```python
from build123d import *

# Parameters (mm, degrees)
SALIENTE_EXTRUIR1_DEPTH = 19.65
CROQUIS2_R              = 2.575
CORTAR_EXTRUIR1_DEPTH   = 8.65


with BuildPart() as part:
    # Croquis1 → Saliente-Extruir1 (new body)
    with BuildSketch(Plane(origin=(0, 0, 0), x_dir=(1, 0, 0), z_dir=(0, 1, 0))):
        with BuildLine():
            Line((-5.5, 9.825), (5.5, 9.825))
            ThreePointArc((5.5, 9.825), (6.207106781, 9.532106781), (6.5, 8.825))
            Line((6.5, 8.825), (6.5, -8.825))
            ThreePointArc((6.5, -8.825), (6.207106781, -9.532106781), (5.5, -9.825))
            Line((5.5, -9.825), (-5.5, -9.825))
            ThreePointArc((-5.5, -9.825), (-6.207106781, -9.532106781), (-6.5, -8.825))
            Line((-6.5, -8.825), (-6.5, 8.825))
            ThreePointArc((-6.5, 8.825), (-6.207106781, 9.532106781), (-5.5, 9.825))
        make_face()
        with BuildLine():
            Line((-4.75, -6.825), (4.75, -6.825))
            ThreePointArc((4.75, -6.825), (4.926776695, -6.751776695), (5, -6.575))
            Line((5, -6.575), (5, 7.325))
            ThreePointArc((5, 7.325), (4.707106781, 8.032106781), (4, 8.325))
            Line((4, 8.325), (-4, 8.325))
            ThreePointArc((-4, 8.325), (-4.707106781, 8.032106781), (-5, 7.325))
            Line((-5, 7.325), (-5, -6.575))
            ThreePointArc((-5, -6.575), (-4.926776695, -6.751776695), (-4.75, -6.825))
        make_face(mode=Mode.SUBTRACT)
    extrude(amount=-SALIENTE_EXTRUIR1_DEPTH)

    # Croquis2 → Cortar-Extruir1 (cut)
    with BuildSketch(Plane.XY.offset(9.825)):
        with Locations((0, -4.65)):
            Circle(CROQUIS2_R)
        with Locations((0, -15)):
            Circle(CROQUIS2_R)
    extrude(amount=-CORTAR_EXTRUIR1_DEPTH, mode=Mode.SUBTRACT)


solid = part.part
```
The listing builds one solid part. Answer for the finished solid, in the listing's coordinates (mm). A direction names the side the tool comes from. Round coordinates to 2 decimals unless told otherwise and drop trailing zeros. Loops run counter-clockwise (first coordinate to the right, second up) from the corner with the lowest first, then second, coordinate; pieces in that order, holes last. Notation, with made-up numbers: (-32.75, 69.25) -> (0.25, 69.25) arc R12 ccw to (0.25, 90.25) -> close; hole circle Ø3 at (15.25, 81). An arc over 180 degrees is marked (long way). Use one line per item in the form item = value.
1. The part is cut by section D-D on y = -15. Determine the outline of the cut face in (x, z) (3 decimals).
Answer key:
outline = (-6.5, -8.825) arc R1 ccw to (-5.5, -9.825) -> (5.5, -9.825) arc R1 ccw to (6.5, -8.825) -> (6.5, 8.825) arc R1 ccw to (5.5, 9.825) -> (2.575, 9.825) -> (2.575, 6.825) -> (4.75, 6.825) arc R0.25 cw to (5, 6.575) -> (5, -7.325) arc R1 cw to (4, -8.325) -> (-4, -8.325) arc R1 cw to (-5, -7.325) -> (-5, 6.575) arc R0.25 cw to (-4.75, 6.825) -> (-2.575, 6.825) -> (-2.575, 9.825) -> (-5.5, 9.825) arc R1 ccw to (-6.5, 8.825) -> close
2. Find the intervals of material crossed by probe 1 along Y at (x, z) = (0, 9.1) (3 decimals); probe 2 along Z at (x, y) = (0.25, -10.5) (3 decimals); probe 3 along X at (y, z) = (-10, 6.5), in increasing order. Write a range as [from, to].
Answer key:
probe_1 = [-19.65, -17.575], [-12.425, -7.225], [-2.075, 0]
probe_2 = [-9.825, -8.325], [6.825, 9.825]
probe_3 = [-6.5, -5], [5, 6.5]
3. For a pull along Z with two mould halves and no side action, classify faces 1 (the cylindrical face through (-6.2, -9.69, 9.54)), 2 (the flat face through (6, 0, 0)), 3 (the flat face through (0, -10, -9.825)), 4 (the cylindrical face through (-4.7, -9.69, -8.04)) as released by +Z, released by -Z, zero draft, split by the parting line, or undercut.
Answer key:
face_1 = released by +Z
face_2 = zero draft
face_3 = released by -Z
face_4 = undercut
4. The part is cut by section B-B on z = 3.75. Determine the outline of the cut face in (x, y).
Answer key:
outline = (-6.5, -19.65) -> (-5, -19.65) -> (-5, 0) -> (-6.5, 0) -> close; (5, -19.65) -> (6.5, -19.65) -> (6.5, 0) -> (5, 0) -> close
5. The part is cut by section A-A on x = -3.25. Determine the outline of the cut face in (y, z) (3 decimals), and give its area (3 significant figures).
Answer key:
outline = (-19.65, -9.825) -> (0, -9.825) -> (0, -8.325) -> (-19.65, -8.325) -> close; (-19.65, 6.825) -> (0, 6.825) -> (0, 9.825) -> (-19.65, 9.825) -> close
area = 88.4 mm²
6. A tool of negligible diameter and unlimited length cuts with its end or side. For faces 5 (the cylindrical face through (-0.558, -7.164, 8.346)), 6 (the flat face through (5, -10, 0)), 7 (the flat face through (6.5, -10, 0)), from which of +Z, -Z, +X, -X, +Y, -Y can it reach the whole face along a straight path? Write none if from no direction.
Answer key:
face_5 = +Z
face_6 = +Y, -Y
face_7 = +Z, -Z, +X, +Y, -Y
7. The part is cut by section C-C on x = 0. Determine the outline of the cut face in (y, z) (3 decimals).
Answer key:
outline = (-19.65, -9.825) -> (0, -9.825) -> (0, -8.325) -> (-19.65, -8.325) -> close; (-19.65, 6.825) -> (-17.575, 6.825) -> (-17.575, 9.825) -> (-19.65, 9.825) -> close; (-12.425, 6.825) -> (-7.225, 6.825) -> (-7.225, 9.825) -> (-12.425, 9.825) -> close; (-2.075, 6.825) -> (0, 6.825) -> (0, 9.825) -> (-2.075, 9.825) -> close
